The drawing under review shows one solid part. Ordinate dimensions are in mm from its lowest x, y, z. A direction names the side the tool comes from. Round coordinates to 2 decimals unless told otherwise and drop trailing zeros. Write each loop counter-clockwise with the first axis right and the second up, starting at its lowest first coordinate (ties: lowest second). Pieces come first, ordered by that corner, then holes.
Item 1: To check wall thickness, follow L1, parallel to Z at x = 25, y = 18; L2, parallel to Y at x = 15.75, z = 26.5 (1 decimal). State the ranges of each line that lie inside material, in increasing order.
Item 2: Clearance check with flat-ended pins moving along their axes: pin 1 Ø2 at (x, y) = (4.5, 4) entering from +Z; pin 2 Ø6 at (x, z) = (15, 24) entering from +Y; pin 3 Ø12 at (y, z) = (16, 26) entering from +X; pin 4 Ø3 at (x, y) = (7.5, 10.5) entering from -Z. State where each tip first meets the part, or that it passes through.
Item 3: Add section A-A (z = 3.5). Give the boundary of the cut face in (x, y) (1 decimal), plus the area to 3 significant figures.
Item 4: Machinability: for the marked faces 1 and 2, which of the approach directions +Z, -Z, +X, -X, +Y, -Y give a long, thin tool a straight path to every point of the face, cutting with its end or side? Answer none if there is none.
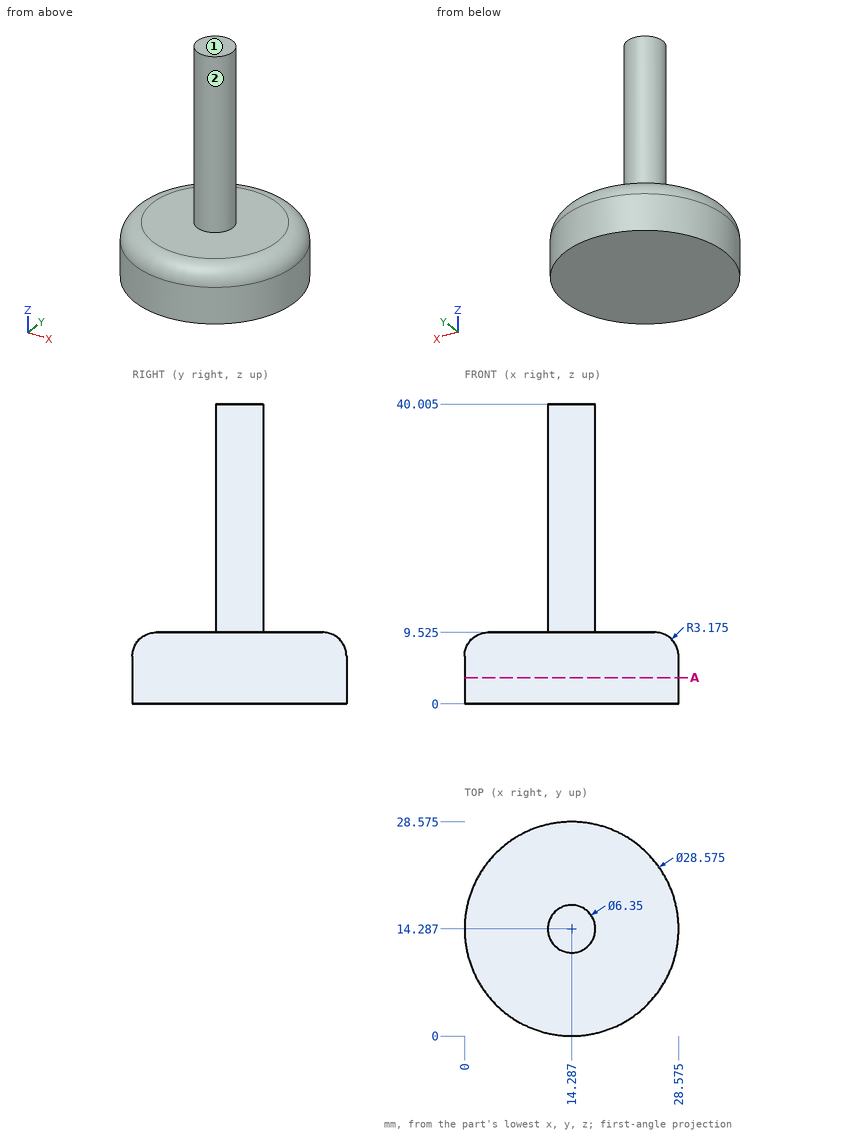
Numbers:
1. L1: z = 0 to 9.52
1. L2: y = 11.5 to 17.1
2. pin 1: stops at z = 8.74
2. pin 2: stops at y = 17.46
2. pin 3: stops at x = 17.46
2. pin 4: stops at z = 0
3. outline: circle Ø28.6 at (14.3, 14.3)
3. area: 641 mm2
4. face 1: +Z, +X, -X, +Y, -Y
4. face 2: +Z
